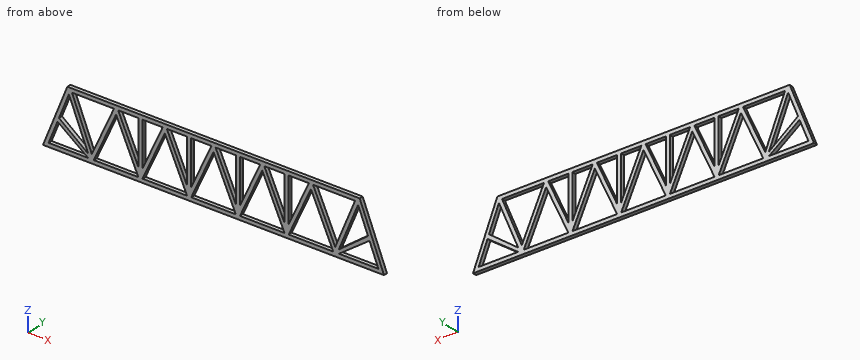
from build123d import *

# Parameters (mm, degrees)
F1_DEPTH = 3.175
F3_W     = 3.175
F3_H     = 50.8
F4_DEPTH = 3.175
F6_DEPTH = 3.175


# Not quite as in the source:
# - a length typed as a fraction of an inch, garbled in the dataset ("3 / 203.2 mm" for 3/8 in), is restored


with BuildPart() as f1:
    # F0 (on Front) → F1 (new body)
    with BuildSketch(Plane.XZ):
        Polygon((-100.2748559753, 0), (0, 0), (0, 3.175), (-18.5744864726, 3.175), (0, 43.8066891587), (0, 47.625), (0, 50.8), (-121.92, 50.8), (-132.0796890642, 25.4007773395), (-140.97, 3.175), (-142.24, 0), align=None)
        Polygon((-104.6410501003, 3.175), (-137.5504203475, 3.175), (-130.1349730994, 21.7136181201), align=None, mode=Mode.SUBTRACT)
        Polygon((-62.7055135274, 3.175), (-99.8544864726, 3.175), (-81.28, 43.8066891587), align=None, mode=Mode.SUBTRACT)
        Polygon((-40.64, 43.8066891587), (-22.0655135274, 3.175), (-59.2144864726, 3.175), align=None, mode=Mode.SUBTRACT)
        Polygon((-128.8950878765, 24.8133311775), (-120.6186164373, 45.5045097755), (-104.527521639, 6.3479696325), align=None, mode=Mode.SUBTRACT)
        Polygon((-101.5186177981, 7.1713344078), (-118.0554031391, 47.625), (-83.0255135274, 47.625), align=None, mode=Mode.SUBTRACT)
        Polygon((-60.96, 6.9933108413), (-79.5344864726, 47.625), (-42.3855135274, 47.625), align=None, mode=Mode.SUBTRACT)
        Polygon((-38.8944864726, 47.625), (-1.7455135274, 47.625), (-20.32, 6.9933108413), align=None, mode=Mode.SUBTRACT)
    extrude(amount=F1_DEPTH)

    # F2: F1 across face


with BuildPart() as f1_1:
    add(f1.part)
    add(f1.part.mirror(Plane(origin=(0, -1.5875, 47.3033445794), x_dir=(0, 1, 0), z_dir=(1, 0, 0))))

    # F3 (on Front) → F4 (join)
    with BuildSketch(Plane.XZ):
        with Locations((-60.96, 25.4)):
            Rectangle(F3_W, F3_H)
        with Locations((-20.32, 25.4)):
            Rectangle(F3_W, F3_H)
        with Locations((60.96, 25.4)):
            Rectangle(F3_W, F3_H)
        Polygon((22.0655135274, 0), (21.9075, 6.9933108413), (21.9075, 50.8), (18.7325, 50.8), (18.7325, 0), align=None)
    extrude(amount=F4_DEPTH)


with BuildPart() as f6:
    # F5 (on Front) → F6 (new body)
    with BuildSketch(Plane.XZ):
        Polygon((14.0807485003, -20.7951998672), (-43.0692514997, -20.7951998672), (-43.0692514997, -23.9701998672), (-39.8942514997, -23.9701998672), (-39.8942514997, -27.1451998672), (10.9057485003, -27.1451998672), (10.9057485003, -23.9701998672), (14.0807485003, -23.9701998672), align=None)
    extrude(amount=F6_DEPTH)


solid = f1_1.part
Work out the finished part from the listing and answer in its coordinate system (mm). Give positions to 0.01 mm unless a question says otherwise; leave off trailing zeros. Loops run counter-clockwise (first coordinate to the right, second up) from the corner with the lowest first, then second, coordinate; pieces in that order, holes last. Notation, with made-up numbers: (-34.5, 43.5) -> (20.5, 43.5) arc R27 ccw to (20.5, 61.5) -> close; hole circle Ø6 at (4, 78). An arc over 180 degrees is marked (long way). Use a Markdown table: item, result. Add a question column.
1) The part is cut by section A-A, the plane x = -88. Determine the outline of the cut face in (y, z) (3 decimals), plus the area to 3 significant figures.
2) Consider line 1 along Z through (x, y) = (46.5, -1.7) (3 decimals); line 2 along Z through (x, y) = (-53, -1.35) (3 decimals); line 3 along Z through (x, y) = (106, -2.45) (3 decimals). Determine where each line is inside the solid, lowest interval first.
3) The part is cut by section B-B, the plane y = -2.55. Count the separate pieces of the cut face and the enclosed holes in it, plus the area to 3 significant figures.
4) Each of these flat-tipped pins is pushed along its axis until it touches: P1, Ø1, axis at y = -2, z = 36.5, coming from the +X side; P2, Ø1.5, axis at y = -2, z = 36.5, coming from the +X side; P3, Ø1, axis at y = -1.5, z = 30, coming from the +X side; P4, Ø5, axis at x = 85.5, z = 23.5, coming from the +Y side. Where does it stop, or does it pass through?
Reported:
| question | item | result |
|---|---|---|
| 1 | outline | (-3.175, 0) -> (0, 0) -> (0, 3.175) -> (-3.175, 3.175) -> close; (-3.175, 29.107) -> (0, 29.107) -> (0, 36.743) -> (-3.175, 36.743) -> close; (-3.175, 47.625) -> (0, 47.625) -> (0, 50.8) -> (-3.175, 50.8) -> close |
| 1 | area | 44.4 mm^2 |
| 2 | line 1 | z = 0 to 3.175, 30.988 to 38.625, 47.625 to 50.8 |
| 2 | line 2 | z = 0 to 3.175, 16.769 to 24.406, 47.625 to 50.8 |
| 2 | line 3 | z = 0 to 3.175, 4.163 to 7.464, 9.931 to 18.134, 47.625 to 50.8 |
| 3 | separate pieces | 1 |
| 3 | enclosed holes | 19 |
| 3 | area | 4,440 mm^2 |
| 4 | P1 | stops at x = 127.84 |
| 4 | P2 | stops at x = 127.94 |
| 4 | P3 | stops at x = 130.44 |
| 4 | P4 | passes through |
